Input: part model. Units: mm. Frame: model coordinates. A direction names the side the tool comes from. Give positions to 0.01 mm unless a question says otherwise; leave off trailing zeros. Loops run counter-clockwise (first coordinate to the right, second up) from the corner with the lowest first, then second, coordinate; pieces in that order, holes last. Notation, with made-up numbers: (-14, 45) - (-6, 45) arc R26 ccw to (-6, 61) - close; hole circle Ø7 at (21, 57). An arc over 180 degrees is marked (long way). Answer as a JSON object with one key per item and string values. Group by question number.
(1) Material intervals for L1, parallel to X at y = -157.5, z = 136; L2, parallel to Y at x = -150.5, z = 157.5; L3, parallel to Y at x = -70.5, z = 202.5, sorted ascending.
(2) Pin query (flat end, axial travel): P1, Ø2, axis at y = -125.5, z = 55.5, coming from the +X side; P2, Ø15.5, axis at x = -27.5, z = 161, coming from the +Y side; P3, Ø1.7, axis at x = -168.5, z = 161, coming from the +Y side. Return the tip coordinate at first contact, or that it passes through.
(3) Access query for faces 1 (the flat face through (-31, -170.18, 161)), 2 (the flat face through (-122, -121, 317.5)). Directions: +Z, -Z, +X, -X, +Y, -Y. A direction counts if a zero-diameter tool reaches every point of the face in a straight line with its end or side. Return the directions, or none.
(4) Section query C-C (x = -51.5). Return loops of the section in (y, z), plus the area to 3 significant figures.
(5) Section query A-A (z = 40.5). Return loops of the section in (x, y), plus the area to 3 significant figures.
(6) Section query B-B (y = -69.5). Return loops of the section in (x, z).
Autodesk Inventor part; units mm, degrees
ref_plane "YZ Plane" through (0, 0, 0) normal (1, 0, 0) x (0, 1, 0)
ref_plane "XZ Plane" through (0, 0, 0) normal (0, 1, 0) x (-1, 0, 0)
ref_plane "XY Plane" through (0, 0, 0) normal (0, 0, 1) x (1, 0, 0)
sketch "Sketch1" plane through (0, 0, 0) normal (0, 0, 1) x (1, 0, 0)
  circle A0 centre (0, 0) radius 177.8
  circle A1 centre (0, 0) radius 171.45
  dimension "d0" = 355.6
  dimension "d1" = 342.9
extrude "Extrusion1" add sketch "Sketch1" along normal blind 317.5
sketch "Sketch2" plane through (0, 0, 317.5) normal (0, 0, 1) x (1, 0, 0)
  circle A0 centre (0, 0) radius 171.45
  circle A1 centre (0, 0) radius 177.8
  line L0 (0, 0) -> (-195.3507, 0)
  line L1 (-170.18, -40) -> (-165.608, -40)
  line L2 (-165.608, -40) -> (-165.608, 40)
  line L3 (-165.608, 40) -> (-170.18, 40)
  line L4 (-170.18, 40) -> (-170.18, -40)
  dimension "d4" = 80
  dimension "d5" = 165.608
  dimension "d6" = 4.572
extrude "Extrusion2" cut sketch "Sketch2" against normal blind 317.5 contours L3 L2 L0 L4 A0 | A0 L4 L3 | L1 L4 A0 | A0 L4 L0 L2 L1
pattern_circular "Circular Pattern1" count 4 over 360 about axis through (0, 0, -10) along (0, 0, 1) of "Extrusion2"
sketch "Sketch3" plane through (0, 0, 317.5) normal (0, 0, 1) x (1, 0, 0)
  line L0 (-205.5346, 0) -> (309.1067, 0)
  line L1 (309.1067, 0) -> (309.1067, 465.2654)
  line L2 (309.1067, 465.2654) -> (-205.5346, 465.2654)
  line L3 (-205.5346, 465.2654) -> (-205.5346, 0)
  line L4 (0, 604.1533) -> (225.7004, 604.1533)
  line L5 (225.7004, 604.1533) -> (225.7004, -403.3158)
  line L6 (225.7004, -403.3158) -> (0, -403.3158)
  line L7 (0, -403.3158) -> (0, 604.1533)
extrude "Extrusion3" cut sketch "Sketch3" against normal blind 317.5
properties part number "skin.25"
Recorded:
{
 "1": {"L1": "x = -82.5 to -67.74", "L2": "y = -94.67 to -82.13", "L3": "y = -163.23 to -156.28"},
 "2": {"P1": "stops at x = -115.73", "P2": "stops at y = -170.18", "P3": "stops at y = -40"},
 "3": {"face 1": "+Z, -Z, +X, +Y", "face 2": "+Z, +X, -X, +Y, -Y"},
 "4": {"outline": "(-170.18, 0) - (-163.53, 0) - (-163.53, 317.5) - (-170.18, 317.5) - close", "area": "2,110 mm^2"},
 "5": {"outline": "(-177.8, 0) arc R177.8 ccw to (0, -177.8) - (0, -171.45) arc R171.45 cw to (-20.83, -170.18) - (-40, -170.18) - (-40, -166.72) arc R171.45 cw to (-166.72, -40) - (-170.18, -40) - (-170.18, -20.83) arc R171.45 cw to (-171.45, 0) - close", "area": "1,680 mm^2"},
 "6": {"outline": "(-163.65, 0) - (-156.73, 0) - (-156.73, 317.5) - (-163.65, 317.5) - close"}
}
